Verification items for the finished model (mm, model axes). Face numbers are marked on the shaded views. A direction names the side the tool comes from. Coordinates: 2 decimals unless noted, no trailing zeros. Loops run counter-clockwise (first coordinate to the right, second up) from the corner with the lowest first, then second, coordinate; pieces in that order, holes last. Notation, with made-up numbers: (-3.75, -28) -> (11.25, -28) arc R30 cw to (11.25, 4) -> close; hole circle Ø1 at (-16.75, -22.5). An arc over 180 degrees is marked (long way). Answer as a JSON object with one key per item and string values. Group by question number.
Q1. Scan lines: L1, parallel to Y at x = 2.75, z = 1.05 (1 decimal); L2, parallel to Y at x = 5.75, z = 0.7 (1 decimal); L3, parallel to X at y = 2, z = 0.3. Record each from-to range of solid material in increasing order.
Q2. Cross-section at D-D on z = 2.4. Record the boundary of the cut face in (x, y) (1 decimal), and give its area (3 significant figures).
Q3. Release check for a two-part mould opening along Y. For the marked faces 3, 4 and 5 record: released by +Y, released by -Y, zero draft, split by the parting line, or undercut.
Q4. Gauge pin test, flat ends, axial feed: pin 1 Ø2.5 at (x, y) = (3.97, -11.91) entering from -Z; pin 2 Ø0.5 at (x, y) = (3.5, 12) entering from -Z (3 decimals); pin 3 Ø1 at (x, y) = (4, -1) entering from +Z (3 decimals). Record the tip position at first contact, or that the pin passes through.
Q5. Cross-section at A-A on z = 0.65. Give the number of separate pieces and of enclosed holes in the cut face, and give its area (3 significant figures).
Q6. Cross-section at C-C on x = 5.75. Record the boundary of the cut face in (y, z) (1 decimal).
Q7. Set-up check for the marked faces 1 and 2: record each of +Z, -Z, +X, -X, +Y, -Y from which the full face is reachable in a straight line by a thin tool's end or side.
```python
from build123d import *

# Parameters (mm, degrees)
F0_R     = 2.38125
F1_DEPTH = 3.175
F2_DEPTH = 4.7625
F3_T     = -1.5875
F4_R     = 3.175
F4_R_2   = 2.38125
F5_DEPTH = 1.5875


with BuildPart() as f1:
    # F0 (on Top) → F1 (new body)
    with BuildSketch(Plane.XY):
        Polygon((7.9375, 15.875), (0, 15.875), (-7.9375, -15.875), (7.9375, -15.875), align=None)
        with Locations((3.96875, -11.90625)):
            Circle(F0_R, mode=Mode.SUBTRACT)
        with Locations((3.96875, -3.96875)):
            Circle(F0_R, mode=Mode.SUBTRACT)
        with Locations((3.96875, 3.96875)):
            Circle(F0_R, mode=Mode.SUBTRACT)
        with Locations((3.96875, 11.90625)):
            Circle(F0_R, mode=Mode.SUBTRACT)
    extrude(amount=F1_DEPTH)

    # F0 (on Top) → F2 (join)
    with BuildSketch(Plane.XY):
        with Locations((3.96875, 11.90625)):
            Circle(F0_R)
        with Locations((3.96875, 3.96875)):
            Circle(F0_R)
        with Locations((3.96875, -3.96875)):
            Circle(F0_R)
        with Locations((3.96875, -11.90625)):
            Circle(F0_R)
    extrude(amount=F2_DEPTH)

    # F3
    f3_openings = [f1.faces().sort_by_distance(p)[0] for p in [
        (1.763889, -1.763889, 0),
    ]]
    offset(amount=F3_T, openings=f3_openings, kind=Kind.INTERSECTION)

    # F4 (on face) → F5 (join)
    with BuildSketch(Plane(origin=(0, 0, 1.5875), x_dir=(1, 0, 0), z_dir=(0, 0, -1))):
        with BuildLine():
            ThreePointArc((0.4381385265, -11.0821239253), (2.3949650124, -10.0219106095), (3.175, -7.9375))
            ThreePointArc((3.175, -7.9375), (1.8179135149, -5.3344603437), (-1.0932302062, -4.9566489946))
            Line((-1.0932302062, -4.9566489946), (-0.8992491716, -5.7325731328))
            ThreePointArc((-0.8992491716, -5.7325731328), (1.3283475585, -5.9611790933), (2.38125, -7.9375))
            ThreePointArc((2.38125, -7.9375), (1.7680146479, -9.5326413001), (0.244157492, -10.3061997871))
            Line((0.244157492, -10.3061997871), (0.4381385265, -11.0821239253))
        make_face()
        with BuildLine():
            Line((-2.0152745824, -1.2684714896), (-1.6550091801, -2.7095330988))
            ThreePointArc((-1.6550091801, -2.7095330988), (1.5533787132, -2.7690503017), (3.175, 0))
            ThreePointArc((3.175, 0), (0.8354053628, 3.0631230599), (-2.7353766172, 1.6119366495))
            Line((-2.7353766172, 1.6119366495), (-2.3751112149, 0.1708750402))
            ThreePointArc((-2.3751112149, 0.1708750402), (0.0854926372, 2.3797148089), (2.38125, 0))
            ThreePointArc((2.38125, 0), (0.6601056594, -2.2879274641), (-2.0152745824, -1.2684714896))
        make_face()
        with Locations((0, 7.9375)):
            Circle(F4_R)
        with Locations((0, 7.9375)):
            Circle(F4_R_2, mode=Mode.SUBTRACT)
    extrude(amount=F5_DEPTH)


solid = f1.part
```
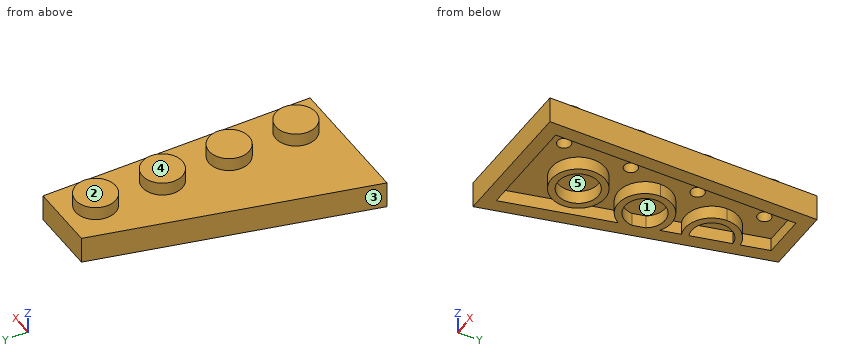
Computed values:
{
 "1": {"L1": "y = -15.9 to -14.3, -9.5 to -6.4, -1.6 to 1.6, 6.4 to 9.5, 14.3 to 15.9", "L2": "y = -15.9 to -14.3, 14.3 to 15.9", "L3": "x = -3.47 to -1.29, 1.29 to 2.47, 6.35 to 7.94"},
 "2": {"outline": "(-7.9, -15.9) -> (7.9, -15.9) -> (7.9, 15.9) -> (0, 15.9) -> close; hole circle Ø1.6 at (4, -11.9); hole circle Ø1.6 at (4, -4); hole circle Ø1.6 at (4, 4); hole circle Ø1.6 at (4, 11.9)", "area": "370 mm²"},
 "3": {"face 3": "released by +Y", "face 4": "zero draft", "face 5": "undercut"},
 "4": {"pin 1": "stops at z = 1.59", "pin 2": "stops at z = 3.175", "pin 3": "stops at z = 3.175"},
 "5": {"separate pieces": "2", "enclosed holes": "4", "area": "162 mm²"},
 "6": {"outline": "(-15.9, 0) -> (-14.3, 0) -> (-14.3, 1.6) -> (14.3, 1.6) -> (14.3, 0) -> (15.9, 0) -> (15.9, 3.2) -> (13.5, 3.2) -> (13.5, 4.8) -> (10.3, 4.8) -> (10.3, 3.2) -> (5.5, 3.2) -> (5.5, 4.8) -> (2.4, 4.8) -> (2.4, 3.2) -> (-2.4, 3.2) -> (-2.4, 4.8) -> (-5.5, 4.8) -> (-5.5, 3.2) -> (-10.3, 3.2) -> (-10.3, 4.8) -> (-13.5, 4.8) -> (-13.5, 3.2) -> (-15.9, 3.2) -> close"},
 "7": {"face 1": "-Z", "face 2": "+Z, +X, -X, +Y, -Y"}
}
